from build123d import *

# Parameters (mm, degrees)
CYLINDER055_R            = 3
CYLINDER055_DEPTH        = 26
CYLINDER047_R            = 1.65
CYLINDER047_DEPTH        = 23
CYLINDER046_R            = 1.65
CYLINDER046_DEPTH        = 23
BOX079_W                 = 3
BOX079_H                 = 17
BOX079_DEPTH             = 20
FILLET005015030019017_R  = 1
BOX080_W                 = 3
BOX080_H                 = 17
BOX080_DEPTH             = 10
CHAMFER010015011014_SIZE = 2
BOX078_W                 = 3
BOX078_H                 = 8
BOX078_DEPTH             = 20
FILLET005015030019016_R  = 1
CYLINDER054_R            = 3.15
CYLINDER054_DEPTH        = 10
BOX082_W                 = 18
BOX082_H                 = 1
BOX082_DEPTH             = 7.8
BOX081_W                 = 18
BOX081_H                 = 5
BOX081_DEPTH             = 16
CHAMFER010015011015_SIZE = 2
CHAMFER010015011016_SIZE = 1


with BuildPart() as cylinder055:
    # Cylinder055 → Cylinder055 (new body)
    with BuildSketch(Plane(origin=(40, 19.5, 6), x_dir=(0, 0, -1), z_dir=(1, 0, 0))):
        Circle(CYLINDER055_R)
    extrude(amount=CYLINDER055_DEPTH)


with BuildPart() as cylinder047:
    # Cylinder047 → Cylinder047 (new body)
    with BuildSketch(Plane(origin=(37, 12.5, 16), x_dir=(0, 0, -1), z_dir=(1, 0, 0))):
        Circle(CYLINDER047_R)
    extrude(amount=CYLINDER047_DEPTH)


with BuildPart() as fusion001021004009015013018008006003:
    # Cylinder046 → Cylinder046 (new body)
    with BuildSketch(Plane(origin=(37, -12.5, 16), x_dir=(0, 0, -1), z_dir=(1, 0, 0))):
        Circle(CYLINDER046_R)
    extrude(amount=CYLINDER046_DEPTH)

    # Fusion001021004009015013018008006003: union Cylinder047
    add(cylinder047.part)


with BuildPart() as fillet005015030019017:
    # Box079 → Box079 (new body)
    with BuildSketch(Plane(origin=(46, 8.5, 0), x_dir=(1, 0, 0), z_dir=(0, 0, 1))):
        with Locations((1.5, 8.5)):
            Rectangle(BOX079_W, BOX079_H)
    extrude(amount=BOX079_DEPTH)

    # Fillet005015030019017
    fillet005015030019017_edges = [fillet005015030019017.edges().sort_by_distance(p)[0] for p in [
        (47.5, 8.5, 20),
        (47.5, 25.5, 0),
    ]]
    fillet(fillet005015030019017_edges, radius=FILLET005015030019017_R)


with BuildPart() as chamfer010015011014:
    # Box080 → Box080 (new body)
    with BuildSketch(Plane(origin=(46, -8.5, 0), x_dir=(1, 0, 0), z_dir=(0, 0, 1))):
        with Locations((1.5, 8.5)):
            Rectangle(BOX080_W, BOX080_H)
    extrude(amount=BOX080_DEPTH)

    # Chamfer010015011014
    chamfer010015011014_edges = [chamfer010015011014.edges().sort_by_distance(p)[0] for p in [
        (49, 0, 10),
    ]]
    chamfer(chamfer010015011014_edges, length=CHAMFER010015011014_SIZE)


with BuildPart() as fillet005015030019016:
    # Box078 → Box078 (new body)
    with BuildSketch(Plane(origin=(46, -16.5, 0), x_dir=(1, 0, 0), z_dir=(0, 0, 1))):
        with Locations((1.5, 4)):
            Rectangle(BOX078_W, BOX078_H)
    extrude(amount=BOX078_DEPTH)

    # Fillet005015030019016
    fillet005015030019016_edges = [fillet005015030019016.edges().sort_by_distance(p)[0] for p in [
        (47.5, -16.5, 0),
        (47.5, -16.5, 20),
        (47.5, -8.5, 20),
    ]]
    fillet(fillet005015030019016_edges, radius=FILLET005015030019016_R)


with BuildPart() as cylinder054:
    # Cylinder054 → Cylinder054 (new body)
    with BuildSketch(Plane(origin=(56.5, 17.5, 14), x_dir=(0, 0, -1), z_dir=(0, 1, 0))):
        Circle(CYLINDER054_R)
    extrude(amount=CYLINDER054_DEPTH)


with BuildPart() as cube080:
    # Box082 → Box082 (new body)
    with BuildSketch(Plane(origin=(46, 25.5, 10.1), x_dir=(1, 0, 0), z_dir=(0, 0, 1))):
        with Locations((9, 0.5)):
            Rectangle(BOX082_W, BOX082_H)
    extrude(amount=BOX082_DEPTH)


with BuildPart() as chamfer010015011016:
    # Box081 → Box081 (new body)
    with BuildSketch(Plane(origin=(46, 20.5, 6), x_dir=(1, 0, 0), z_dir=(0, 0, 1))):
        with Locations((9, 2.5)):
            Rectangle(BOX081_W, BOX081_H)
    extrude(amount=BOX081_DEPTH)

    # Chamfer010015011015
    chamfer010015011015_edges = [chamfer010015011016.edges().sort_by_distance(p)[0] for p in [
        (46, 23, 22),
        (64, 23, 22),
        (64, 23, 6),
    ]]
    chamfer(chamfer010015011015_edges, length=CHAMFER010015011015_SIZE)

    # Fusion001021004009015013018008006004: union Cube080
    add(cube080.part)

    # Cut019003010005001012: cut Cylinder054
    add(cylinder054.part, mode=Mode.SUBTRACT)

    # Fusion001021004009015013018008006005: union Fillet005015030019017, Chamfer010015011014, Fillet005015030019016
    add(fillet005015030019017.part)
    add(chamfer010015011014.part)
    add(fillet005015030019016.part)

    # Cut019003010005001013: cut Fusion001021004009015013018008006003
    add(fusion001021004009015013018008006003.part, mode=Mode.SUBTRACT)

    # Cut019003010005001014: cut Cylinder055
    add(cylinder055.part, mode=Mode.SUBTRACT)

    # Chamfer010015011016
    chamfer010015011016_edges = [chamfer010015011016.edges().sort_by_distance(p)[0] for p in [
        (49, 16.543204, 6.507306),
    ]]
    chamfer(chamfer010015011016_edges, length=CHAMFER010015011016_SIZE)


solid = chamfer010015011016.part
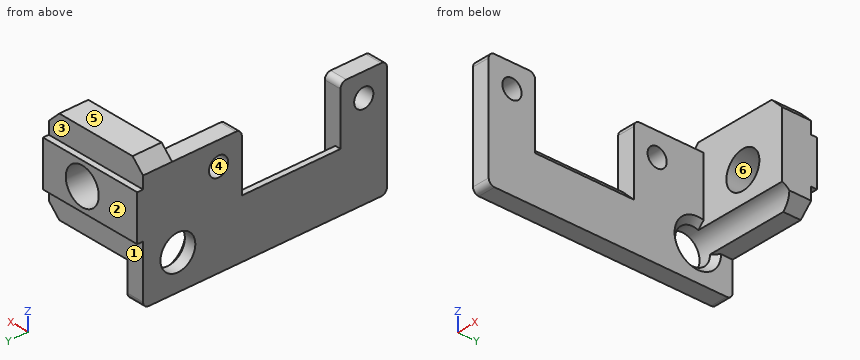
Read the model definition and answer for the solid it produces. Units are mm, in the model's axes. Face numbers are marked on the shaded views. A direction names the side the tool comes from. Coordinates: 2 decimals unless noted, no trailing zeros. Write each loop counter-clockwise with the first axis right and the second up, starting at its lowest first coordinate (ties: lowest second). Pieces come first, ordered by that corner, then holes. Notation, with made-up numbers: (55.5, 45) -> (71.5, 45) arc R28 ccw to (71.5, 84) -> close; hole circle Ø9 at (0, 45). An arc over 180 degrees is marked (long way). Return JSON: item names as keys, results as strings.
(1) Each of these flat-tipped pins is pushed along its axis until it touches: P1, Ø4, axis at x = 56.5, z = 14, coming from the +Y side; P2, Ø6, axis at y = -5.5, z = 10, coming from the +X side; P3, Ø10, axis at x = 48.5, y = 1.5, coming from the +Z side; P4, Ø2.5, axis at x = 48, y = -11.5, coming from the +Z side. Where does it stop, or does it pass through?
Answers below:
{"P1": "through", "P2": "x = 49", "P3": "z = 10", "P4": "z = 20"}
(2) The part is cut by section A-A on y = 12.5. Give the vertices of the cut face in (x, z), then the cut area to 3 significant figures.
Answers below:
{"outline": "(46, 0) -> (49, 0) -> (49, 14.35) -> (46, 14.35) -> close; (46, 17.65) -> (49, 17.65) -> (49, 20) -> (46, 20) -> close", "area": "50.1 mm^2"}
(3) Consider line 1 along Y through (x, z) = (47.05, 16); line 2 along Z through (x, y) = (46.9, 12.5); line 3 along Y through (x, z) = (57, 20.25). Determine where each line is inside the solid, lowest interval first. Write a range as from..to.
Answers below:
{"line 1": "-16.5..-14.15, -10.85..-8.5, 8.5..10.85, 14.15..26.5", "line 2": "0..14.35, 17.65..20", "line 3": "20.5..25.5"}
(4) The part is cut by section C-C on z = 16. Give the vertices of the cut face in (x, y).
Answers below:
{"outline": "(46, -16.5) -> (49, -16.5) -> (49, -14.15) -> (46, -14.15) -> close; (46, -10.85) -> (49, -10.85) -> (49, -8.5) -> (46, -8.5) -> close; (46, 8.5) -> (49, 8.5) -> (49, 10.85) -> (46, 10.85) -> close; (46, 14.15) -> (49, 14.15) -> (49, 20.5) -> (54.07, 20.5) -> (54.07, 26.5) -> (46, 26.5) -> close; (58.93, 20.5) -> (64, 20.5) -> (64, 26.5) -> (58.93, 26.5) -> close"}
(5) The part is cut by section B-B on x = 47.5. Give the vertices of the cut face in (y, z).
Answers below:
{"outline": "(-16.5, 1) arc R1 ccw to (-15.5, 0) -> (24.5, 0) arc R1 ccw to (25.5, 1) -> (25.5, 10.1) -> (26.5, 10.1) -> (26.5, 17.9) -> (25.5, 17.9) -> (25.5, 21.5) -> (20.5, 21.5) -> (20.5, 20) -> (9.5, 20) arc R1 ccw to (8.5, 19) -> (8.5, 9.5) -> (-8.5, 9.5) -> (-8.5, 19) arc R1 ccw to (-9.5, 20) -> (-15.5, 20) arc R1 ccw to (-16.5, 19) -> close; hole circle Ø3.3 at (-12.5, 16); hole circle Ø3.3 at (12.5, 16); hole circle Ø6 at (19.5, 6)"}
(6) The part is cut by section D-D on x = 56.5. Give the vertices of the cut face in (y, z), then the cut area to 3 significant figures.
Answers below:
{"outline": "(20.5, 8.83) arc R3 cw to (22.5, 6) -> (25.5, 6) -> (25.5, 10.1) -> (26.5, 10.1) -> (26.5, 10.85) -> (20.5, 10.85) -> close; (20.5, 17.15) -> (26.5, 17.15) -> (26.5, 17.9) -> (25.5, 17.9) -> (25.5, 22) -> (20.5, 22) -> close", "area": "45.9 mm^2"}
(7) Which of the six approach directions +Z, -Z, +X, -X, +Y, -Y give full straight-line access (tool end or side, diameter ignored) to the marked faces 1 and 2?
Answers below:
{"face 1": "-Z, +X, -X, +Y", "face 2": "+Z, -Z, +X, -X, +Y"}
(8) For a pull along Z with two mould halves and no side action, classify the marked faces 3, 4, 5 and 6 as pulls with the +Z half, pulls with the -Z half, needs draft (parallel to the pull), parting line crosses it, or undercut.
Answers below:
{"face 3": "needs draft", "face 4": "undercut", "face 5": "pulls with the +Z half", "face 6": "undercut"}
